Verification items for the finished model (mm, model axes). A direction names the side the tool comes from. Coordinates: 2 decimals unless noted, no trailing zeros. Loops run counter-clockwise (first coordinate to the right, second up) from the corner with the lowest first, then second, coordinate; pieces in that order, holes last. Notation, with made-up numbers: M 47.25,32 L 76.25,32 A11 cw 76.25,38 Z; hole C -21.75,86.5 d8. An arc over 180 degrees is marked long. Write item = value, one per line. Start each with the question number.
```python
from build123d import *

# Parameters (mm, degrees)
EXTRUDE_3_DEPTH    = 3
SKETCH1_W          = 15
SKETCH1_H          = 40
SKETCH1_W_2        = 3
SKETCH1_H_2        = 20
CUT_EXTRUDE1_DEPTH = 10


with BuildPart() as part:
    # Эскиз4 → Бобышка-Вытянуть3 (new body)
    with BuildSketch(Plane(origin=(0, 0, 0), x_dir=(1, 0, 0), z_dir=(0, 1, 0))):
        Polygon((78, 0), (78, 110), (58, 110), (58, 107), (55, 107), (52, 107), (52, 110), (0, 110), (0, 58), (3, 58), (3, 55), (3, 52), (0, 52), (0, 0), (52, 0), (52, 3), (55, 3), (58, 3), (58, 0), align=None)
    extrude(amount=EXTRUDE_3_DEPTH)

    # Sketch1 → Cut-Extrude1 (cut)
    with BuildSketch(Plane(origin=(0, 3, 0), x_dir=(1, 0, 0), z_dir=(0, 1, 0))):
        with Locations((26.5, 55)):
            Rectangle(SKETCH1_W, SKETCH1_H)
        with Locations((55, 55)):
            Rectangle(SKETCH1_W_2, SKETCH1_H_2)
    extrude(amount=-CUT_EXTRUDE1_DEPTH, mode=Mode.SUBTRACT)


solid = part.part
```
Q1. Sectioned sample at B-B on y = 0.9. Record the cut outline in (x, z).
Q2. Set-up check for faces 4 (the face through (3, 1, -55)), 5 (the face through (55, 2, -65)), 6 (the face through (52, 1, -1)), 7 (the face through (26, 1, 0)), 8 (the face through (58, 1, -109)): record each of +Z, -Z, +X, -X, +Y, -Y from which the full face is reachable in a straight line by a thin tool's end or side.
Q3. Mould release check, pull along Z, two halves, no side actions. Record for faces 1 (the face through (26, 2, -75)), 2 (the face through (68, 1, -110)), 3 (the face through (0, 1, -84)): +Z half, -Z half, draft (parallel to the pull), parting line (faces both ways), or undercut.
Q4. Sectioned sample at A-A on z = -62.5. Record the cut outline in (x, y), plus the area to 3 significant figures.
Q5. Sectioned sample at D-D on z = -42. Record the cut outline in (x, y), plus the area to 3 significant figures.
Q6. Scan lines: L1, parallel to X at y = 0.4, z = -64.5; L2, parallel to X at y = 2.55, z = -55; L3, parallel to X at y = 0.4, z = -74. Record each from-to range of solid material in increasing order. Write a range as [from, to].
Q7. Sectioned sample at C-C on x = 20.5. Record the cut outline in (y, z).
Q8. Gauge pin test, flat ends, axial feed: pin 1 (1.5 mm diameter, centred on y = 2, z = -55.5, fed in from -X); pin 2 (1.5 mm diameter, centred on x = 56, y = 2, fed in from +Z); pin 3 (1.5 mm diameter, centred on x = 53.5, y = 1.5, fed in from -Z). Record the tip position at first contact, or that the pin passes through.
Solutions:
q1.outline = M 0,-110 L 52,-110 L 52,-107 L 58,-107 L 58,-110 L 78,-110 L 78,0 L 58,0 L 58,-3 L 52,-3 L 52,0 L 0,0 L 0,-52 L 3,-52 L 3,-58 L 0,-58 Z; hole M 19,-75 L 34,-75 L 34,-35 L 19,-35 Z; hole M 53.5,-65 L 56.5,-65 L 56.5,-45 L 53.5,-45 Z
q2.face_4 = -X, +Y, -Y
q2.face_5 = +Y, -Y
q2.face_6 = +Z, +Y, -Y
q2.face_7 = +Z, +X, -X, +Y, -Y
q2.face_8 = -Z, +Y, -Y
q3.face_1 = undercut
q3.face_2 = -Z half
q3.face_3 = draft
q4.outline = M 0,0 L 19,0 L 19,3 L 0,3 Z; M 34,0 L 53.5,0 L 53.5,3 L 34,3 Z; M 56.5,0 L 78,0 L 78,3 L 56.5,3 Z
q4.area = 180 mm²
q5.outline = M 0,0 L 19,0 L 19,3 L 0,3 Z; M 34,0 L 78,0 L 78,3 L 34,3 Z
q5.area = 189 mm²
q6.L1 = [0, 19], [34, 53.5], [56.5, 78]
q6.L2 = [3, 19], [34, 53.5], [56.5, 78]
q6.L3 = [0, 19], [34, 78]
q7.outline = M 0,-110 L 3,-110 L 3,-75 L 0,-75 Z; M 0,-35 L 3,-35 L 3,0 L 0,0 Z
q8.pin_1 = 3
q8.pin_2 = -3
q8.pin_3 = -107
